from build123d import *

# Parameters (mm, degrees)
F1_DEPTH = 38.1
F2_R     = 5.08
F3_R     = 12.7


with BuildPart() as f1:
    # F0 (on Front) → F1 (new body)
    with BuildSketch(Plane.XZ):
        Polygon((47.388378, -28.077184), (35.071938, 41.772816), (-35.071938, 41.772816), (-47.388378, -28.077184), (-56.209706, -78.105418), (-46.829412, -79.759417), (-46.537767, -78.105418), (-39.395954, -37.602184), (-37.71644, -28.077184), (-27.079514, 32.247816), (27.079514, 32.247816), (37.71644, -28.077184), (39.395954, -37.602184), (46.537767, -78.105418), (46.829412, -79.759417), (56.209706, -78.105418), align=None)
    extrude(amount=F1_DEPTH)

    # F2
    f2_edges = [f1.edges().sort_by_distance(p)[0] for p in [
        (-27.079514, -19.05, 32.247816),
        (27.079514, -19.05, 32.247816),
    ]]
    fillet(f2_edges, radius=F2_R)

    # F3
    f3_edges = [f1.edges().sort_by_distance(p)[0] for p in [
        (-35.071938, -19.05, 41.772816),
        (35.071938, -19.05, 41.772816),
    ]]
    fillet(f3_edges, radius=F3_R)


solid = f1.part
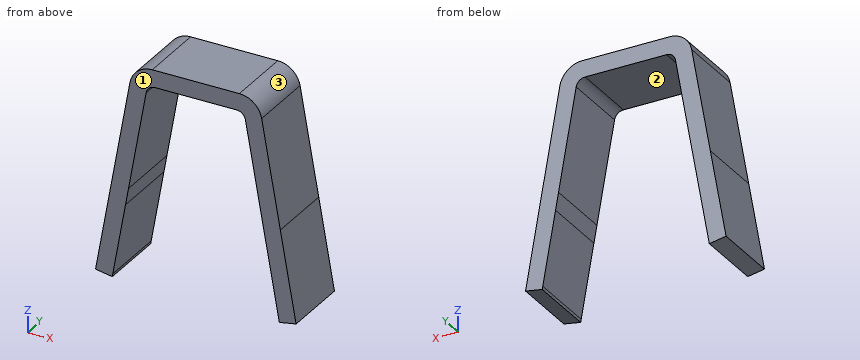
The listing builds one solid part. Answer for the finished solid, in the listing's coordinates (mm). Face numbers are marked on the shaded views. Give positions to 0.01 mm unless a question says otherwise; leave off trailing zeros. Loops run counter-clockwise (first coordinate to the right, second up) from the corner with the lowest first, then second, coordinate; pieces in that order, holes last.
Item 1: A cutting plane is placed at C-C (x = 8). Give the vertices of the cut face in (y, z), then the cut area to 3 significant figures.
Derived:
outline: (-38.1, 32.25) - (0, 32.25) - (0, 41.77) - (-38.1, 41.77) - close
area: 363 mm2
Item 2: Each of these flat-tipped pins is pushed along its axis until it touches: pin 1 Ø4 at (y, z) = (-13.5, -12) entering from -X; pin 2 Ø11.5 at (x, y) = (1.5, -17) entering from -Z. Where does it stop, or does it pass through?
Derived:
pin 1: stops at x = -44.91
pin 2: stops at z = 32.25
Item 3: A cutting plane is placed at B-B (y = -24). Give the vertices of the cut face in (x, z).
Derived:
outline: (-56.21, -78.11) - (-46.83, -79.76) - (-46.54, -78.11) - (-27.82, 28.05) arc R5.08 cw to (-22.82, 32.25) - (22.82, 32.25) arc R5.08 cw to (27.82, 28.05) - (46.54, -78.11) - (46.83, -79.76) - (56.21, -78.11) - (36.92, 31.28) arc R12.7 ccw to (24.42, 41.77) - (-24.42, 41.77) arc R12.7 ccw to (-36.92, 31.28) - close
Item 4: A cutting plane is placed at D-D (x = -34). Give the vertices of the cut face in (y, z).
Derived:
outline: (-38.1, -7) - (0, -7) - (0, 37.4) - (-38.1, 37.4) - close
Item 5: A cutting plane is placed at A-A (z = 3.5). Give the vertices of the cut face in (x, y), then the cut area to 3 significant figures.
Derived:
outline: (-41.82, -38.1) - (-32.15, -38.1) - (-32.15, 0) - (-41.82, 0) - close; (32.15, -38.1) - (41.82, -38.1) - (41.82, 0) - (32.15, 0) - close
area: 737 mm2
Item 6: Determine the mould class of the marked faces 1, 2 and 3 for opening direction X: +X half, -X half, draft (parallel to the pull), parting line (faces both ways), or undercut.
Derived:
face 1: draft
face 2: undercut
face 3: +X half
Item 7: Find the intervals of material crossed by line 1 along X through (y, z) = (-4, 25); line 2 along X through (y, z) = (-7.5, -11); line 3 along Z through (x, y) = (6.5, -14), in increasing order.
Derived:
line 1: x = -38.03 to -28.36, 28.36 to 38.03
line 2: x = -44.38 to -34.71, 34.71 to 44.38
line 3: z = 32.25 to 41.77
